```python
from build123d import *

# Parameters (mm, degrees)
F1_DEPTH = 25.4


with BuildPart() as f1:
    # F0 (on Front) → F1 (new body)
    with BuildSketch(Plane.XZ):
        with BuildLine():
            Line((47.452234, -9.261301), (47.452234, 6.77889))
            Line((47.452234, 6.77889), (16.51758, 6.77889))
            Line((16.51758, 6.77889), (10.788937, 6.77889))
            ThreePointArc((10.788937, 6.77889), (-0.65962, 1.80786), (-11.934666, 7.160799))
            Line((-11.934666, 7.160799), (-17.663306, 7.160799))
            Line((-17.663306, 7.160799), (-48.216049, 7.160799))
            Line((-48.216049, 7.160799), (-48.216049, -9.261301))
            Line((-48.216049, -9.261301), (-42.869318, -9.261301))
            ThreePointArc((-42.869318, -9.261301), (-33.417064, -4.032086), (-23.964809, -9.261301))
            Line((-23.964809, -9.261301), (23.582902, -9.261301))
            ThreePointArc((23.582902, -9.261301), (32.366816, -4.289359), (41.15073, -9.261301))
            Line((41.15073, -9.261301), (47.452234, -9.261301))
        make_face()
        with BuildLine():
            ThreePointArc((23.582902, -9.261301), (32.366816, -17.508878), (41.15073, -9.261301))
            ThreePointArc((41.15073, -9.261301), (32.366816, -4.289359), (23.582902, -9.261301))
        make_face()
        with BuildLine():
            ThreePointArc((-42.869318, -9.261301), (-33.417064, -17.845475), (-23.964809, -9.261301))
            ThreePointArc((-23.964809, -9.261301), (-33.417064, -4.032086), (-42.869318, -9.261301))
        make_face()
    extrude(amount=F1_DEPTH)


solid = f1.part
```
Check sheet for the modelled part. Datum: model origin and axes. Units: mm. A direction names the side the tool comes from. Round coordinates to 2 decimals unless told otherwise and drop trailing zeros. Order: outer loops, then holes, each group sorted by start corner. A loop starts at its lowest first (then second) coordinate and runs counter-clockwise, first axis right, second up.
1) Section check B-B (y = -22.5). Record the boundary of the cut face in (x, z).
2) Go/stop test with flat-tipped pins: pin 1 Ø7.5 at (x, y) = (29.5, -12.5) entering from +Z; pin 2 Ø7.5 at (x, y) = (-1.5, -10) entering from -Z; pin 3 Ø4 at (y, z) = (-12, -14.5) entering from -X. Record where each tip stops, or that it passes through.
3) Section check A-A (z = -14.75). Record the boundary of the cut face in (x, y), and give its area (3 significant figures).
4) Section check D-D (x = -41.5). Record the boundary of the cut face in (y, z), and give its area (3 significant figures).
5) Tool access check on faces 4 (the flat face through (-46, -13, -9.261)), 5 (the flat face through (-1, -13, -9.261)), 6 (the flat face through (29, -13, 6.779)). Record the directions out of +Z, -Z, +X, -X, +Y, -Y that give a thin tool (end or side, any length) a straight path to the whole face; none if there is none.
6) Section check C-C (x = -20.5). Record the boundary of the cut face in (y, z), and give its area (3 significant figures).
7) Scan lines: line 1 (Z direction, x = -12, y = -17.5); line 2 (X direction, y = -23.5, z = -16.25); line 3 (Z direction, x = 42, y = -18.25). Record each from-to range of solid material in increasing order.
8) Mould release check, pull along X, two halves, no side actions. Record for faces 1 (the flat face through (-48.216, -13, -1)), 2 (the cylindrical face through (32.181, -12.522, -17.507)), 3 (the flat face through (44, -13, -9.261)): +X half, -X half, draft (parallel to the pull), parting line (faces both ways), or undercut.
Result:
1. outline: (-48.22, -9.26) - (-42.87, -9.26) arc R9.5 ccw to (-23.96, -9.26) - (23.58, -9.26) arc R8.8 ccw to (41.15, -9.26) - (47.45, -9.26) - (47.45, 6.78) - (10.79, 6.78) arc R15.09 cw to (-11.93, 7.16) - (-48.22, 7.16) - close
2. pin 1: stops at z = 6.78
2. pin 2: stops at z = -9.26
2. pin 3: stops at x = -41.96
3. outline: (-40.43, -25.4) - (-26.4, -25.4) - (-26.4, 0) - (-40.43, 0) - close; (25.97, -25.4) - (38.77, -25.4) - (38.77, 0) - (25.97, 0) - close
3. area: 681 mm2
4. outline: (-25.4, -13.33) - (0, -13.33) - (0, 7.16) - (-25.4, 7.16) - close
4. area: 521 mm2
5. face 4: -Z, -X, +Y, -Y
5. face 5: -Z, +Y, -Y
5. face 6: +Z, +X, +Y, -Y
6. outline: (-25.4, -9.26) - (0, -9.26) - (0, 7.16) - (-25.4, 7.16) - close
6. area: 417 mm2
7. line 1: z = -9.26 to 7.16
7. line 2: x = -38.69 to -28.15, 27.83 to 36.9
7. line 3: z = -9.26 to 6.78
8. face 1: -X half
8. face 2: undercut
8. face 3: draft
